Part print with two shaded views. Sizes in mm from the minimum x, y, z corner. Round coordinates to 2 decimals unless told otherwise and drop trailing zeros. Loops run counter-clockwise (first coordinate to the right, second up) from the corner with the lowest first, then second, coordinate; pieces in that order, holes last.
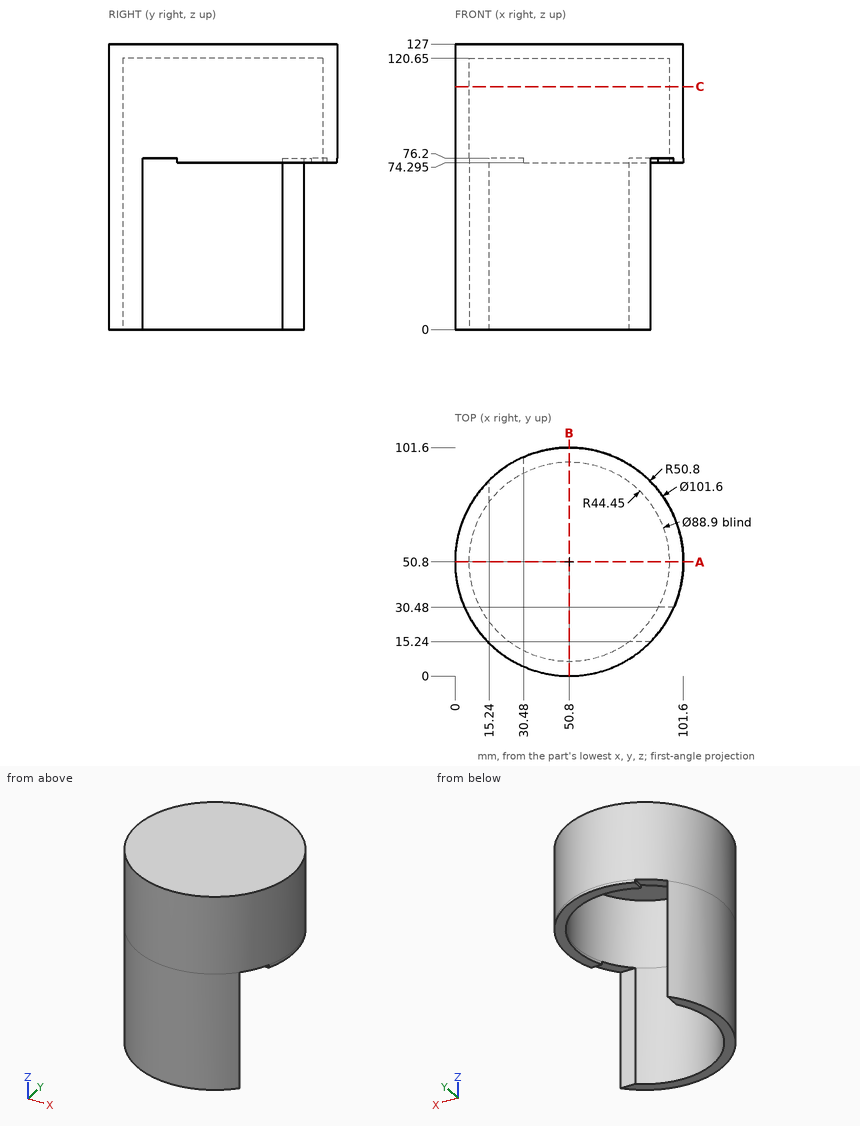
Item 1: Wall check: L1, parallel to Y at x = 50, z = 103; L2, parallel to X at y = 50.8, z = 86; L3, parallel to Z at x = 36, y = 54. Give the ranges that are in metal, low to high.
Verdict:
L1: y = 0.01 to 6.36, 95.24 to 101.59
L2: x = 0 to 6.35, 95.25 to 101.6
L3: z = 120.65 to 127
Item 2: Cut at C-C (z = 108). List the corners of the cut face in (x, y).
Verdict:
outline: circle Ø101.6 at (50.8, 50.8); hole circle Ø88.9 at (50.8, 50.8)
Item 3: Flat gauge pins, fed straight in: P1, Ø2, axis at x = 49.5, y = 62, coming from the -Z side; P2, Ø7.5, axis at x = 22.5, y = 85.5, coming from the -Z side; P3, Ø1.5, axis at x = 55.5, z = 39, coming from the +Y side. Where does each tip first touch, or does it go through?
Verdict:
P1: stops at z = 120.65
P2: stops at z = 76.2
P3: stops at y = 6.69
Item 4: Cut at A-A (y = 50.8). List the corners of the cut face in (x, z) (3 decimals).
Verdict:
outline: (0, 0) - (6.35, 0) - (6.35, 120.65) - (95.25, 120.65) - (95.25, 74.295) - (101.6, 74.295) - (101.6, 127) - (0, 127) - close
